The listing builds one solid part. Answer for the finished solid, in the listing's coordinates (mm). Face numbers are marked on the shaded views. A direction names the side the tool comes from. Coordinates: 2 decimals unless noted, no trailing zeros. Loops run counter-clockwise (first coordinate to the right, second up) from the corner with the lowest first, then second, coordinate; pieces in that order, holes last. Notation, with made-up numbers: M 83.5,-18.75 L 129.5,-18.75 A36 cw 129.5,17.25 Z; hole C -4,17 d4. An arc over 180 degrees is marked long. Answer as a JSON object with one key per item and string values. Group by question number.
1. Given pin 1 (18.5 mm diameter, centred on x = -100, y = 12, fed in from -Z); pin 2 (2 mm diameter, centred on x = -40.5, y = 3, fed in from -Z); pin 3 (18.5 mm diameter, centred on y = 27.5, z = 6, fed in from +X), each flat-ended and moving along its own axis, determine where each tip first touches the part or whether it passes through.
2. A cutting plane is placed at D-D on x = -19.5. Give the vertices of the cut face in (y, z).
3. A cutting plane is placed at B-B on x = -66.5. Give the vertices of the cut face in (y, z).
4. For the marked faces 1, 2 and 3, determine the directions among +Z, -Z, +X, -X, +Y, -Y from which every point of the face is accessible in a straight line to the end or side of a thin tool.
5. Straight lines are drawn through the part: L1, parallel to Z at x = -61, y = 3; L2, parallel to Y at x = -11, z = -7; L3, parallel to Z at x = -103, y = 46. For each, find the intervals that lie inside material, in ascending order.
6. A cutting plane is placed at C-C on y = 30. Give the vertices of the cut face in (x, z), and give its area (3 significant figures).
7. A cutting plane is placed at A-A on z = 8. Give the vertices of the cut face in (x, y).
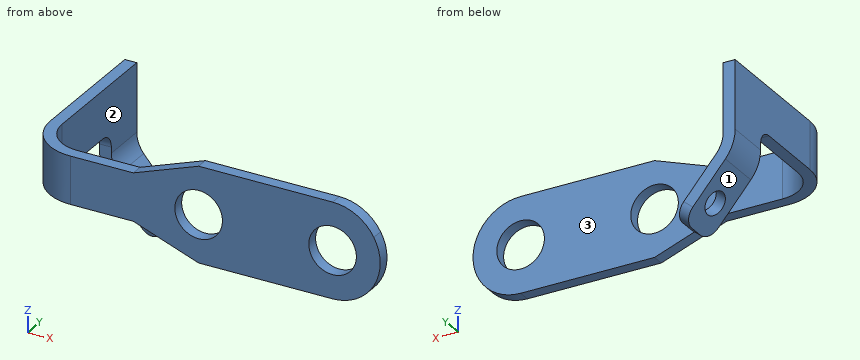
from build123d import *

# Parameters (mm, degrees)
EXTRUDE_THIN1_DEPTH     = 16
SKETCH2_R               = 20
SKETCH2_R_2             = 16
CUT_EXTRUDE_THIN1_DEPTH = 10
BOSS_EXTRUDE1_DEPTH     = 4
SKETCH2_6_R             = 8
CUT_EXTRUDE1_DEPTH      = 4
EXTRUDE_THIN2_DEPTH     = 15
FILLET1_R               = 5
FILLET2_R               = 5
SKETCH5_R               = 4
CUT_EXTRUDE2_DEPTH      = 15


with BuildPart() as part:
    # Sketch1 → Extrude-Thin1 (new body)
    with BuildSketch(Plane.XY):
        with BuildLine():
            Line((0, 0), (-104, 0))
            ThreePointArc((-104, 0), (-115.313708499, 4.686291501), (-120, 16))
            Line((-120, 16), (-120, 60))
            Line((-120, 60), (-116, 60))
            Line((-116, 60), (-116, 16))
            ThreePointArc((-116, 16), (-112.485281374, 7.514718626), (-104, 4))
            Line((-104, 4), (0, 4))
            Line((0, 4), (0, 0))
        make_face()
    extrude(amount=EXTRUDE_THIN1_DEPTH)

    # Sketch2 → Cut-Extrude-Thin1 (cut)
    with BuildSketch(Plane(origin=(0, 4, 0), x_dir=(1, 0, 0), z_dir=(0, 1, 0))):
        with Locations((-16, -8)):
            Circle(SKETCH2_R)
        with Locations((-16, -8)):
            Circle(SKETCH2_R_2, mode=Mode.SUBTRACT)
    extrude(amount=-CUT_EXTRUDE_THIN1_DEPTH, mode=Mode.SUBTRACT)


with BuildPart() as cut_extrude_thin1_piece_1:
    # of the separate pieces the step leaves, piece 1, a body of its own (cut_extrude_thin1_pieces)
    add(part.part.solids().sort_by_distance((-104, 4, 0))[0])



with BuildPart() as cut_extrude_thin1_piece_2:
    # of the separate pieces the step leaves, piece 2, a body of its own (cut_extrude_thin1_pieces)
    add(part.part.solids().sort_by_distance((-29.856406461, 4, 0))[0])


with BuildPart() as cut_extrude_thin1_piece_1_1:
    add(cut_extrude_thin1_piece_1.part)

    add(cut_extrude_thin1_piece_2.part)  # Boss-Extrude1 merges Cut-Extrude-Thin1 piece 2
    # Sketch2_5 → Boss-Extrude1 (add)
    with BuildSketch(Plane(origin=(0, 4, 0), x_dir=(1, 0, 0), z_dir=(0, 1, 0))):
        with BuildLine():
            ThreePointArc((-29.856406461, 0), (-24, 5.856406461), (-16, 8))
            Line((-16, 8), (-61, 8))
            Line((-61, 8), (-82.979819356, 0))
            Line((-82.979819356, 0), (-61, 0))
            Line((-61, 0), (-29.856406461, 0))
        make_face()
        with BuildLine():
            ThreePointArc((-16, -24), (-24, -21.856406461), (-29.856406461, -16))
            Line((-29.856406461, -16), (-61, -16))
            Line((-61, -16), (-82.979819356, -16))
            Line((-82.979819356, -16), (-61, -24))
            Line((-61, -24), (-16, -24))
        make_face()
        with BuildLine():
            ThreePointArc((-29.856406461, -16), (-32, -8), (-29.856406461, 0))
            Line((-29.856406461, 0), (-61, 0))
            ThreePointArc((-61, 0), (-55.343145751, -2.343145751), (-53, -8))
            ThreePointArc((-53, -8), (-55.343145751, -13.656854249), (-61, -16))
            Line((-61, -16), (-29.856406461, -16))
        make_face()
        with BuildLine():
            Line((-16.000000062, -16), (-29.856406461, -16))
            ThreePointArc((-29.856406461, -16), (-24, -21.856406461), (-16, -24))
            ThreePointArc((-16, -24), (-8, -21.856406461), (-2.143593539, -16))
            Line((-2.143593539, -16), (-16.000000062, -16))
        make_face()
        with BuildLine():
            ThreePointArc((-2.143593539, 0), (-8, 5.856406461), (-16, 8))
            ThreePointArc((-16, 8), (-24, 5.856406461), (-29.856406461, 0))
            Line((-29.856406461, 0), (-16, 0))
            Line((-16, 0), (-2.143593539, 0))
        make_face()
        with BuildLine():
            ThreePointArc((0, -8), (-0.545186779, -3.858895278), (-2.143593539, 0))
            Line((-2.143593539, 0), (-16, 0))
            ThreePointArc((-16, 0), (-10.343145751, -2.343145751), (-8, -8))
            ThreePointArc((-8, -8), (-10.343145773, -13.656854272), (-16.000000062, -16))
            Line((-16.000000062, -16), (-2.143593539, -16))
            ThreePointArc((-2.143593539, -16), (-0.545186779, -12.141104722), (0, -8))
        make_face()
        with BuildLine():
            Line((-16, 0), (-29.856406461, 0))
            ThreePointArc((-29.856406461, 0), (-32, -8), (-29.856406461, -16))
            Line((-29.856406461, -16), (-16.000000062, -16))
            ThreePointArc((-16.000000062, -16), (-24, -7.999999969), (-16, 0))
        make_face()
    extrude(amount=-BOSS_EXTRUDE1_DEPTH)

    # Sketch2_6 → Cut-Extrude1 (cut)
    with BuildSketch(Plane(origin=(0, 4, 0), x_dir=(1, 0, 0), z_dir=(0, 1, 0))):
        with Locations(Location((-61, -8, 0), (0, 0, 180))):
            Circle(SKETCH2_6_R)
        with Locations(Location((-16, -8, 0), (0, 0, 180))):
            Circle(SKETCH2_6_R)
    extrude(amount=-CUT_EXTRUDE1_DEPTH, mode=Mode.SUBTRACT)

    # Sketch3 → Extrude-Thin2 (add)
    with BuildSketch(Plane(origin=(0, 60, 0), x_dir=(1, 0, 0), z_dir=(0, 1, 0))):
        with BuildLine():
            Line((-116, 0), (-116, 7))
            ThreePointArc((-116, 7), (-115.396926208, 10.420201433), (-113.660444431, 13.427876097))
            Line((-113.660444431, 13.427876097), (-99.519117018, 30.280853845))
            Line((-99.519117018, 30.280853845), (-102.583294791, 32.852004284))
            Line((-102.583294791, 32.852004284), (-116.724622204, 15.999026536))
            ThreePointArc((-116.724622204, 15.999026536), (-119.155696691, 11.788282007), (-120, 7))
            Line((-120, 7), (-120, 0))
            Line((-120, 0), (-116, 0))
        make_face()
    extrude(amount=-EXTRUDE_THIN2_DEPTH)

    # Fillet1
    fillet1_edges = [cut_extrude_thin1_piece_1_1.edges().sort_by_distance(p)[0] for p in [
        (-118, 45, 0),
    ]]
    fillet(fillet1_edges, radius=FILLET1_R)

    # Fillet2
    fillet2_edges = [cut_extrude_thin1_piece_1_1.edges().sort_by_distance(p)[0] for p in [
        (-101.051205904, 60, -31.566429065),
        (-101.051205904, 45, -31.566429065),
    ]]
    fillet(fillet2_edges, radius=FILLET2_R)

    # Sketch5 → Cut-Extrude2 (cut)
    with BuildSketch(Plane(origin=(-73.310624983, 0, -61.514918385), x_dir=(0.6427876096865427, 0, -0.7660444431189752), z_dir=(0.7660444431189752, 0, 0.6427876096865427))):
        with Locations((-50.773175525, 52.5)):
            Circle(SKETCH5_R)
    extrude(amount=-CUT_EXTRUDE2_DEPTH, mode=Mode.SUBTRACT)


solid = cut_extrude_thin1_piece_1_1.part
From the geometry:
{
 "1": {"pin 1": "stops at z = 0", "pin 2": "stops at z = -8", "pin 3": "stops at x = -116"},
 "2": {"outline": "M 0,-8 L 4,-8 L 4,0.81 L 0,0.81 Z; M 0,15.19 L 4,15.19 L 4,24 L 0,24 Z"},
 "3": {"outline": "M 0,-6 L 4,-6 L 4,2.19 L 0,2.19 Z; M 0,13.81 L 4,13.81 L 4,22 L 0,22 Z"},
 "4": {"face 1": "-Z, -X, +Y, -Y", "face 2": "+Z, +X, +Y", "face 3": "+Z, -Z, +X, +Y"},
 "5": {"L1": "z = -8 to 0, 16 to 24", "L2": "y = 0 to 4", "L3": "z = -30.59 to -26.13"},
 "6": {"outline": "M -120,0 L -116,0 L -116,16 L -120,16 Z", "area": "64.0 mm²"},
 "7": {"outline": "M -120,16 A16 ccw -104,0 L -69,0 L -69,4 L -104,4 A12 cw -116,16 L -116,60 L -120,60 Z; M -53,0 L -24,0 L -24,4 L -53,4 Z; M -8,0 L 0,0 L 0,4 L -8,4 Z"}
}
